Here's how the part is built. I have some questions about the finished solid (model axes, mm). A direction names the side the tool comes from. Round coordinates to 2 decimals unless told otherwise and drop trailing zeros. Write each loop counter-clockwise with the first axis right and the second up, starting at its lowest first coordinate (ties: lowest second). Pieces come first, ordered by that corner, then holes. Notation, with made-up numbers: (-16, 6) - (30, 6) arc R32 ccw to (30, 43) - close; hole circle Ø8 at (-22.75, 56.25). An arc over 180 degrees is marked (long way). Return JSON: item names as keys, results as strings. Group by question number.
```python
from build123d import *

# Parameters (mm, degrees)
BOSS_EXTRUDE1_DEPTH = 38.1
CUT_EXTRUDE1_REACH  = 5.175
SKETCH2_R           = 1.5875
CUT_EXTRUDE2_REACH  = 5.175
SKETCH3_R           = 1.5875


with BuildPart() as part:
    # Sketch1 → Boss-Extrude1 (new body)
    with BuildSketch(Plane(origin=(0, 0, 0), x_dir=(0, 0, -1), z_dir=(1, 0, 0))):
        Polygon((0, 0), (0, 50.8), (3.175, 50.8), (3.175, 3.175), (25.4, 3.175), (25.4, 0), align=None)
    extrude(amount=BOSS_EXTRUDE1_DEPTH)

    # Sketch2 → Cut-Extrude1 (cut, up to next)
    with BuildSketch(Plane(origin=(0, 3.175, 0), x_dir=(1, 0, 0), z_dir=(0, 1, 0)), mode=Mode.PRIVATE) as cut_extrude1_sk1:
        with Locations((28.575, 14.2875)):
            Circle(SKETCH2_R)
    cut_extrude1_tool1 = extrude(cut_extrude1_sk1.sketch, amount=-CUT_EXTRUDE1_REACH, mode=Mode.PRIVATE) & part.part
    add(cut_extrude1_tool1.solids().sort_by_distance((28.575, 3.175, -14.2875))[0], mode=Mode.SUBTRACT)
    # Sketch2 → Cut-Extrude1 (cut, up to next)
    with BuildSketch(Plane(origin=(0, 3.175, 0), x_dir=(1, 0, 0), z_dir=(0, 1, 0)), mode=Mode.PRIVATE) as cut_extrude1_sk2:
        with Locations((9.525, 14.2875)):
            Circle(SKETCH2_R)
    cut_extrude1_tool2 = extrude(cut_extrude1_sk2.sketch, amount=-CUT_EXTRUDE1_REACH, mode=Mode.PRIVATE) & part.part
    add(cut_extrude1_tool2.solids().sort_by_distance((9.525, 3.175, -14.2875))[0], mode=Mode.SUBTRACT)

    # Sketch3 → Cut-Extrude2 (cut, up to next)
    with BuildSketch(Plane(origin=(0, 0, -3.175), x_dir=(-1, 0, 0), z_dir=(0, 0, -1)), mode=Mode.PRIVATE) as cut_extrude2_sk1:
        with Locations((-18.983298196, 12.7)):
            Circle(SKETCH3_R)
    cut_extrude2_tool1 = extrude(cut_extrude2_sk1.sketch, amount=-CUT_EXTRUDE2_REACH, mode=Mode.PRIVATE) & part.part
    add(cut_extrude2_tool1.solids().sort_by_distance((18.983298, 12.7, -3.175))[0], mode=Mode.SUBTRACT)
    # Sketch3 → Cut-Extrude2 (cut, up to next)
    with BuildSketch(Plane(origin=(0, 0, -3.175), x_dir=(-1, 0, 0), z_dir=(0, 0, -1)), mode=Mode.PRIVATE) as cut_extrude2_sk2:
        with Locations((-18.983298196, 41.275)):
            Circle(SKETCH3_R)
    cut_extrude2_tool2 = extrude(cut_extrude2_sk2.sketch, amount=-CUT_EXTRUDE2_REACH, mode=Mode.PRIVATE) & part.part
    add(cut_extrude2_tool2.solids().sort_by_distance((18.983298, 41.275, -3.175))[0], mode=Mode.SUBTRACT)


solid = part.part
```
1) Imagine slicing it at D-D (z = -6). Please give me the cut outline in (x, y) (3 decimals), plus the area to 3 significant figures.
2) Imagine slicing it at C-C (x = 16). Please give me the cut outline in (y, z) (3 decimals), plus the area to 3 significant figures.
3) Imagine slicing it at A-A (y = 12.7). Please give me the cut outline in (x, z) (3 decimals), plus the area to 3 significant figures.
4) Imagine slicing it at B-B (x = 10.5). Please give me the cut outline in (y, z) (3 decimals).
5) I need wall thicknesses on line 1 along Y through (x, z) = (11, -3.5) (3 decimals); line 2 along Z through (x, y) = (33.5, 19.5) (3 decimals). Which ranges of each line are inside material? Lowest first, please.
6) Will these pins go through, and if not, where does the flat tip stop? pin 1 Ø1 at (x, y) = (28, 42) entering from -Z (3 decimals); pin 2 Ø6.5 at (x, z) = (10, -18) entering from +Y (3 decimals).
7) If we mould it in two halves opening along Y, with no side actions, what happens to faces 3 (the flat face through (19, 2, -25.4)), 4 (the flat face through (19, 50.8, -2)), 5 (the cylindrical face through (19.327, 39.725, -1.61))? For each: released by +Y, released by -Y, zero draft, split by the parting line, or undercut.
8) For faces 1 (the flat face through (19, 27, -3.175)), 2 (the cylindrical face through (8.265, 1.61, -13.322)), which set-ups out of +Z, -Z, +X, -X, +Y, -Y let a thin tool reach every point of the face, with its end or its side?
Results found:
{
 "1": {"outline": "(0, 0) - (38.1, 0) - (38.1, 3.175) - (0, 3.175) - close", "area": "121 mm²"},
 "2": {"outline": "(0, -25.4) - (3.175, -25.4) - (3.175, -3.175) - (50.8, -3.175) - (50.8, 0) - (0, 0) - close", "area": "232 mm²"},
 "3": {"outline": "(0, -3.175) - (17.396, -3.175) - (17.396, 0) - (0, 0) - close; (20.571, -3.175) - (38.1, -3.175) - (38.1, 0) - (20.571, 0) - close", "area": "111 mm²"},
 "4": {"outline": "(0, -25.4) - (3.175, -25.4) - (3.175, -15.54) - (0, -15.54) - close; (0, -13.035) - (3.175, -13.035) - (3.175, -3.175) - (50.8, -3.175) - (50.8, 0) - (0, 0) - close"},
 "5": {"line 1": "y = 0 to 3.175", "line 2": "z = -3.175 to 0"},
 "6": {"pin 1": "stops at z = -3.175", "pin 2": "stops at y = 3.175"},
 "7": {"face 3": "zero draft", "face 4": "released by +Y", "face 5": "undercut"},
 "8": {"face 1": "-Z, +X, -X, +Y", "face 2": "+Y, -Y"}
}
